Model file for the job. Use its own axes, mm. Give positions to 0.01 mm unless a question says otherwise; leave off trailing zeros. Answer as a JSON object with one key per item and string values. Group by question number.
```python
from build123d import *

# Parameters (mm, degrees)
SKETCH_1_R      = 2.5
EXTRUDE_1_DEPTH = 1000


with BuildPart() as part:
    # 草图1 → 凸台-拉伸1 (new body)
    with BuildSketch(Plane.XY):
        with BuildLine():
            Line((4.215995631, 3.129161171), (6.436655803, 5.349821343))
            Line((6.436655803, 5.349821343), (7.776655803, 5.349821343))
            ThreePointArc((7.776655803, 5.349821343), (7.988787838, 5.261953377), (8.076655803, 5.049821343))
            Line((8.076655803, 5.049821343), (8.076655803, 3.249821343))
            ThreePointArc((8.076655803, 3.249821343), (8.164523769, 3.037689308), (8.376655803, 2.949821343))
            Line((8.376655803, 2.949821343), (9.376655803, 2.949821343))
            Line((9.376655803, 2.949821343), (9.376655803, 3.249821343))
            ThreePointArc((9.376655803, 3.249821343), (9.435234447, 3.391242699), (9.576655803, 3.449821343))
            Line((9.576655803, 3.449821343), (9.99208048, 3.449821343))
            Line((9.99208048, 3.449821343), (9.99208048, 8.46524602))
            ThreePointArc((9.99208048, 8.46524602), (9.552740652, 9.525906191), (8.49208048, 9.96524602))
            ThreePointArc((8.49208048, 9.96524602), (-4.671012544, 4.512914366), (-10.123344197, -8.650178657))
            ThreePointArc((-10.123344197, -8.650178657), (-9.684004369, -9.710838829), (-8.623344197, -10.150178657))
            Line((-8.623344197, -10.150178657), (-3.723344197, -10.150178657))
            Line((-3.723344197, -10.150178657), (-3.723344197, -9.850178657))
            ThreePointArc((-3.723344197, -9.850178657), (-3.664765553, -9.708757301), (-3.523344197, -9.650178657))
            Line((-3.523344197, -9.650178657), (-3.223344197, -9.650178657))
            Line((-3.223344197, -9.650178657), (-3.223344197, -8.650178657))
            ThreePointArc((-3.223344197, -8.650178657), (-3.311212162, -8.438046623), (-3.523344197, -8.350178657))
            Line((-3.523344197, -8.350178657), (-5.323344197, -8.350178657))
            ThreePointArc((-5.323344197, -8.350178657), (-5.535476231, -8.262310692), (-5.623344197, -8.050178657))
            Line((-5.623344197, -8.050178657), (-5.623344197, -6.710178657))
            Line((-5.623344197, -6.710178657), (-3.402684025, -4.489518485))
            ThreePointArc((-3.402684025, -4.489518485), (-2.916049002, -4.164359358), (-2.342023853, -4.050178657))
            Line((-2.342023853, -4.050178657), (2.09533546, -4.050178657))
            ThreePointArc((2.09533546, -4.050178657), (2.669360608, -4.164359358), (3.155995631, -4.489518485))
            Line((3.155995631, -4.489518485), (5.376655803, -6.710178657))
            Line((5.376655803, -6.710178657), (5.376655803, -8.050178657))
            ThreePointArc((5.376655803, -8.050178657), (5.288787838, -8.262310692), (5.076655803, -8.350178657))
            Line((5.076655803, -8.350178657), (3.276655803, -8.350178657))
            ThreePointArc((3.276655803, -8.350178657), (3.064523769, -8.438046623), (2.976655803, -8.650178657))
            Line((2.976655803, -8.650178657), (2.976655803, -9.650178657))
            Line((2.976655803, -9.650178657), (3.276655803, -9.650178657))
            ThreePointArc((3.276655803, -9.650178657), (3.418077159, -9.708757301), (3.476655803, -9.850178657))
            Line((3.476655803, -9.850178657), (3.476655803, -10.150178657))
            Line((3.476655803, -10.150178657), (8.376655803, -10.150178657))
            ThreePointArc((8.376655803, -10.150178657), (9.437315975, -9.710838829), (9.876655803, -8.650178657))
            Line((9.876655803, -8.650178657), (9.876655803, -3.750178657))
            Line((9.876655803, -3.750178657), (9.576655803, -3.750178657))
            ThreePointArc((9.576655803, -3.750178657), (9.435234447, -3.691600013), (9.376655803, -3.550178657))
            Line((9.376655803, -3.550178657), (9.376655803, -3.250178657))
            Line((9.376655803, -3.250178657), (8.376655803, -3.250178657))
            ThreePointArc((8.376655803, -3.250178657), (8.164523769, -3.338046623), (8.076655803, -3.550178657))
            Line((8.076655803, -3.550178657), (8.076655803, -5.350178657))
            ThreePointArc((8.076655803, -5.350178657), (7.988787838, -5.562310692), (7.776655803, -5.650178657))
            Line((7.776655803, -5.650178657), (6.436655803, -5.650178657))
            Line((6.436655803, -5.650178657), (4.215995631, -3.429518485))
            ThreePointArc((4.215995631, -3.429518485), (3.890836504, -2.942883462), (3.776655803, -2.368858314))
            Line((3.776655803, -2.368858314), (3.776655803, 2.068500999))
            ThreePointArc((3.776655803, 2.068500999), (3.890836504, 2.642526148), (4.215995631, 3.129161171))
        make_face()
        with Locations((-0.123344197, -0.035109627)):
            Circle(SKETCH_1_R, mode=Mode.SUBTRACT)
        with BuildLine():
            Line((5.376655803, 7.864890373), (5.376655803, 6.524890373))
            Line((5.376655803, 6.524890373), (3.155995631, 4.304230202))
            ThreePointArc((3.155995631, 4.304230202), (2.669360608, 3.979071075), (2.09533546, 3.864890373))
            Line((2.09533546, 3.864890373), (-2.342023853, 3.864890373))
            ThreePointArc((-2.342023853, 3.864890373), (-2.69419221, 3.906817176), (-3.026673509, 4.030253775))
            ThreePointArc((-3.026673509, 4.030253775), (0.896523465, 6.557813899), (5.376655803, 7.864890373))
        make_face(mode=Mode.SUBTRACT)
        with BuildLine():
            Line((-4.023344197, 2.18357003), (-4.023344197, -2.253789283))
            ThreePointArc((-4.023344197, -2.253789283), (-4.137524898, -2.827814432), (-4.462684025, -3.314449455))
            Line((-4.462684025, -3.314449455), (-6.683344197, -5.535109627))
            Line((-6.683344197, -5.535109627), (-8.023344197, -5.535109627))
            ThreePointArc((-8.023344197, -5.535109627), (-8.235476231, -5.447241661), (-8.323344197, -5.235109627))
            ThreePointArc((-8.323344197, -5.235109627), (-6.845791054, -0.874365796), (-4.203440462, 2.89620888))
            ThreePointArc((-4.203440462, 2.89620888), (-4.069065062, 2.551091728), (-4.023344197, 2.18357003))
        make_face(mode=Mode.SUBTRACT)
    extrude(amount=EXTRUDE_1_DEPTH)


solid = part.part
```
Q1. Slice it at A-A, the plane z = 621. Count the separate pieces of the cut face and the enclosed holes in it, then the cut area to 3 significant figures.
Q2. Wall check: L1, parallel to Y at x = -4.75, z = 800.5; L2, parallel to Y at x = -4.25, z = 230; L3, parallel to X at y = -0.5, z = 423. Give the ranges that are in metal, low to high.
Q3. Drop flat-ended pins along their axis: P1, Ø1.1, axis at y = -9, z = 486, coming from the +X side; P2, Ø0.7, axis at y = -7.5, z = 615.5, coming from the -X side; P3, Ø6, axis at y = -0.5, z = 584.5, coming from the +X side. Give the stop position or say it passes through.
Solved:
{
 "1": {"separate pieces": "1", "enclosed holes": "3", "area": "166 mm²"},
 "2": {"L1": "y = -10.15 to -8.35, -5.84 to -3.6, 2.28 to 4.43", "L2": "y = -10.15 to -8.35, -5.34 to -3.05, 2.85 to 4.92", "L3": "x = -8.24 to -6.65, -4.02 to -2.58, 2.33 to 3.78"},
 "3": {"P1": "stops at x = 9.88", "P2": "stops at x = -10.11", "P3": "stops at x = 9.38"}
}
